from build123d import *

# Parameters (mm, degrees)
BOSS_EXTRUDE1_DEPTH     = 265
CUT_EXTRUDE2_DEPTH      = 267.364412037
CUT_EXTRUDE2_DEPTH_BACK = 267.364412037
SKETCH3_R               = 7.5
SCALE1_SCALE            = 0.25


with BuildPart() as part:
    # Sketch2 → Boss-Extrude1 (new, symmetric)
    with BuildSketch(Plane(origin=(0, 0, 0), x_dir=(0, 0, -1), z_dir=(1, 0, 0))):
        Polygon((-10, -20), (-10, -25), (10, -25), (10, 25), (-10, 25), (-10, 20), (-7, 21.732050808), (-7, 12.267949192), (-10, 14), (-10, -14), (-7, -12.267949192), (-7, -21.732050808), align=None)
    extrude(amount=BOSS_EXTRUDE1_DEPTH, both=True)

    # Sketch3 → Cut-Extrude2 (cut, two sides: drawn at the far end of the back side and taken through both)
    with BuildSketch(Plane.XY.offset(-CUT_EXTRUDE2_DEPTH_BACK)):
        Circle(SKETCH3_R)
    extrude(amount=CUT_EXTRUDE2_DEPTH + CUT_EXTRUDE2_DEPTH_BACK, mode=Mode.SUBTRACT)


with BuildPart() as part_1:
    # Scale1: scaled about (0, 0, -0.410943417)
    add(part.part.scale(SCALE1_SCALE).moved(Location((0, 0, -0.308207563))))


solid = part_1.part
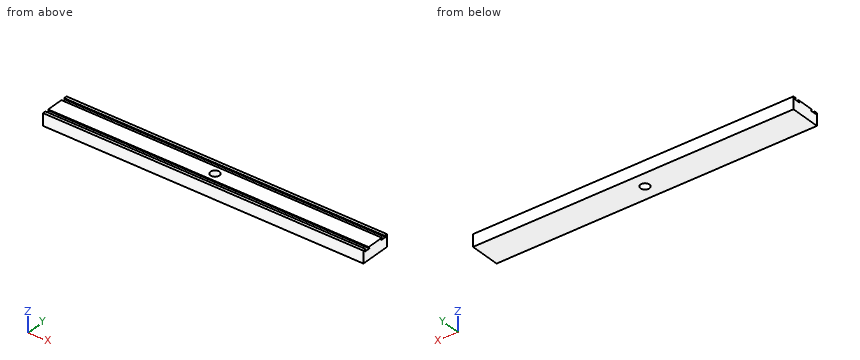
For this review, take the finished solid that the model builds, in its own axes (mm). Round coordinates to 2 decimals unless told otherwise and drop trailing zeros. Write each loop counter-clockwise with the first axis right and the second up, starting at its lowest first coordinate (ties: lowest second). Pieces come first, ordered by that corner, then holes. Notation, with made-up numbers: M -29,72 L -16,72 A19 ccw -16,98 Z; hole C 16,65.5 d7. An arc over 180 degrees is marked long. Write item = value, one per line. Start each with the question number.
(1) We need section B-B (x = 0). Give the boundary of the cut face in (y, z) (3 decimals), then the cut area to 3 significant figures.
(2) We need section A-A (y = 0). Give the boundary of the cut face in (x, z) (3 decimals).
(3) We need section C-C (x = 49.5). Give the boundary of the cut face in (y, z).
(4) For line 1 along Y through (x, z) = (0, -0.6) (3 decimals); line 2 along Y through (x, z) = (-26, 2.05); line 3 along X through (y, z) = (0, 0.1) (3 decimals), list the stretches that pass through material, from the lowest coordinate up.
(5) Clearance check with flat-ended pins moving along their axes: pin 1 Ø4 at (x, y) = (31, -4) entering from +Z; pin 2 Ø0.7 at (x, y) = (-31.5, -4.5) entering from +Z. State where each tip first meets the part, or that it passes through.
Results found:
q1.outline = M -6.25,-2.808 L -1.875,-2.808 L -1.875,2.192 L -3.5,2.192 L -3.067,1.442 L -5.433,1.442 L -5,2.192 L -6.25,2.192 Z; M 1.875,-2.808 L 6.25,-2.808 L 6.25,2.192 L 5,2.192 L 5.433,1.442 L 3.067,1.442 L 3.5,2.192 L 1.875,2.192 Z
q1.area = 40.9 mm²
q2.outline = M -66.25,-2.808 L -1.875,-2.808 L -1.875,2.192 L -66.25,2.192 Z; M 1.875,-2.808 L 66.25,-2.808 L 66.25,2.192 L 1.875,2.192 Z
q3.outline = M -6.25,-2.81 L 6.25,-2.81 L 6.25,2.19 L 5,2.19 L 5.43,1.44 L 3.07,1.44 L 3.5,2.19 L -3.5,2.19 L -3.07,1.44 L -5.43,1.44 L -5,2.19 L -6.25,2.19 Z
q4.line_1 = -6.25 to -1.875, 1.875 to 6.25
q4.line_2 = -6.25 to -5.08, -3.42 to 3.42, 5.08 to 6.25
q4.line_3 = -66.25 to -1.875, 1.875 to 66.25
q5.pin_1 = 2.19
q5.pin_2 = 1.44
